Can you work these out from the model? Positions are in its coordinate system, mm. A direction names the side the tool comes from. Give positions to 0.01 mm unless a question says otherwise; leave off trailing zeros. Order: outer loops, then holes, each group sorted by start corner. A loop starts at its lowest first (then second) coordinate and runs counter-clockwise, first axis right, second up.
Item 1: I want a section at D-D, the plane y = 7.5. Write out the boundary of the cut face in (x, z).
Item 2: If we mould it in two halves opening along X, with no side actions, what happens to faces 3 (the flat face through (63.5, -12, 0)), 4 (the flat face through (31, -50.8, 0)), 5 (the flat face through (25.146, -1, -11))? For each: +X half, -X half, draft (parallel to the pull), parting line (faces both ways), or undercut.
Item 3: I'm going to push flat-ended pins straight in: pin 1 Ø8 at (y, z) = (-35.5, 13) entering from -X; pin 2 Ø20.5 at (x, y) = (40, -14.5) entering from -Z. Where does each tip first touch, or does it pass through?
Item 4: I want a section at B-B, the plane z = -5. Write out the boundary of the cut face in (x, y).
Item 5: If I drill on line 1 along X through (y, z) = (-16, -10); line 2 along Z through (x, y) = (38.5, -42); line 3 along Z through (x, y) = (31, 37), over which ranges is the centre line in solid material (lowest first)?
Item 6: Which directions (+Z, -Z, +X, -X, +Y, -Y) give clear straight access to the entire face, cutting with the end or side of a thin tool? Please do faces 1 (the flat face through (0, -12, 0)), 2 (the flat face through (50.8, -1, -11)).
Item 7: I want a section at A-A, the plane y = 34.5. Write out the boundary of the cut face in (x, z).
Item 8: I want a section at C-C, the plane x = 48.5. Write out the boundary of the cut face in (y, z), then the cut area to 3 significant figures.
```python
from build123d import *

# Parameters (mm, degrees)
F1_DEPTH      = 63.5
F2_W          = 25.654
F2_H          = 16.9195546743
F3_DEPTH      = 50.801
F3_DEPTH_BACK = 50.801


with BuildPart() as f1:
    # F0 (on Right) → F1 (new body)
    with BuildSketch(Plane.YZ):
        Polygon((25.4, 19.05), (-50.8, 19.05), (-50.8, -19.05), (50.8, -19.05), align=None)
    extrude(amount=F1_DEPTH)

    # F2 (on Front) → F3 (cut, two sides)
    with BuildSketch(Plane.XZ) as f3_sk:
        with Locations((37.973, -10.5902226629)):
            Rectangle(F2_W, F2_H)
    extrude(amount=-F3_DEPTH, mode=Mode.SUBTRACT)
    extrude(f3_sk.sketch, amount=F3_DEPTH_BACK, mode=Mode.SUBTRACT)


solid = f1.part
```
Results list:
1. outline: (0, -19.05) - (25.15, -19.05) - (25.15, -2.13) - (50.8, -2.13) - (50.8, -19.05) - (63.5, -19.05) - (63.5, 19.05) - (0, 19.05) - close
2. face 3: +X half
2. face 4: draft
2. face 5: undercut
3. pin 1: stops at x = 0
3. pin 2: stops at z = -2.13
4. outline: (0, -50.8) - (25.15, -50.8) - (25.15, 41.43) - (0, 41.43) - close; (50.8, -50.8) - (63.5, -50.8) - (63.5, 41.43) - (50.8, 41.43) - close
5. line 1: x = 0 to 25.15, 50.8 to 63.5
5. line 2: z = -2.13 to 19.05
5. line 3: z = -2.13 to 1.65
6. face 1: +Z, -Z, -X, +Y, -Y
6. face 2: -Z, +Y, -Y
7. outline: (0, -19.05) - (25.15, -19.05) - (25.15, -2.13) - (50.8, -2.13) - (50.8, -19.05) - (63.5, -19.05) - (63.5, 5.4) - (0, 5.4) - close
8. outline: (-50.8, -2.13) - (39.52, -2.13) - (25.4, 19.05) - (-50.8, 19.05) - close
8. area: 1,760 mm2
